Design review of the part shown in the three views and the two pictorial views. Dimensions are in mm from the part's minimum x, y and z. Round coordinates to 2 decimals unless told otherwise and drop trailing zeros. Order: outer loops, then holes, each group sorted by start corner. A loop starts at its lowest first (then second) coordinate and runs counter-clockwise, first axis right, second up.
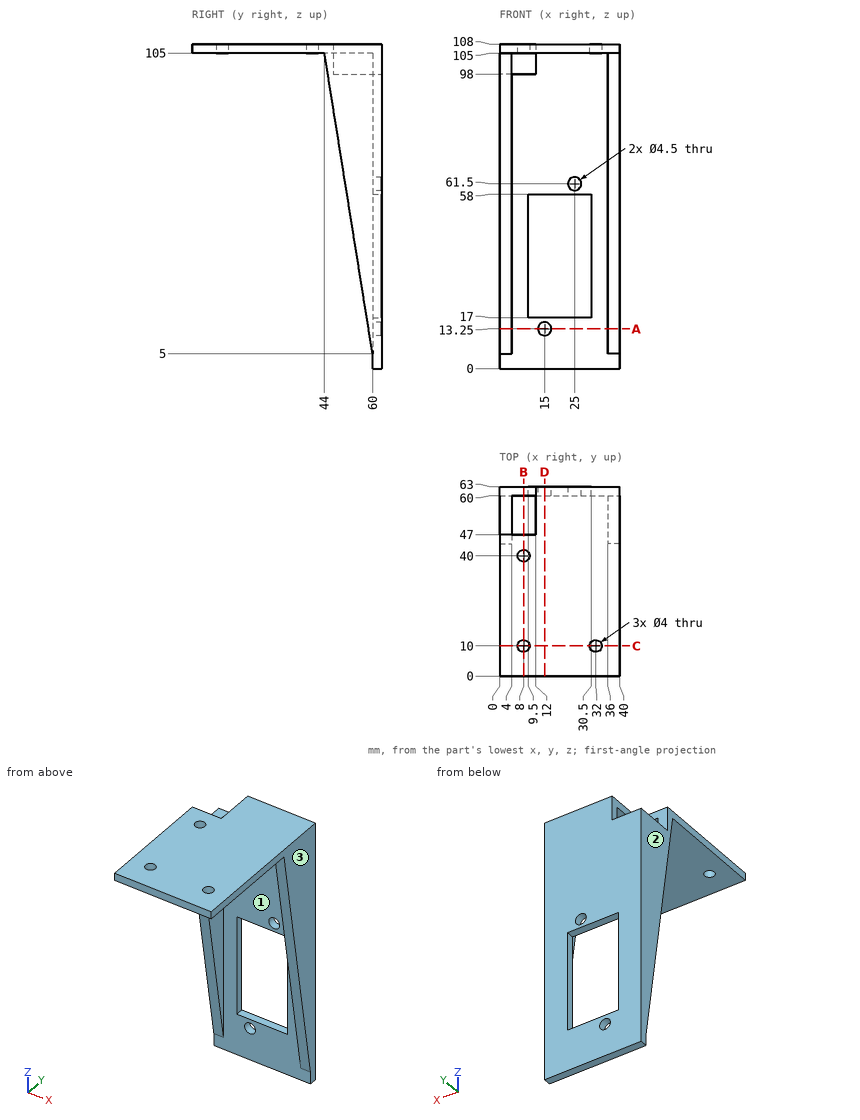
(1) Clearance check with flat-ended pins moving along their axes: P1, Ø3, axis at x = 31, z = 20.5, coming from the -Y side; P2, Ø3, axis at y = 57.5, z = 101, coming from the -X side; P3, Ø11, axis at x = 5.5, z = 104, coming from the +Y side; P4, Ø2.5, axis at x = 25, z = 61.5, coming from the +Y side. State where each tip first meets the part, or that it passes through.
(2) Add section B-B on x = 8. Give the boundary of the cut face in (y, z).
(3) Add section D-D on x = 15. Give the boundary of the cut face in (y, z), plus the area to 4 significant figures.
(4) Draft analysis for pull direction X (two halves, no side actions). For the marked faces 1, 2 and 3, state which applies: pulls with the +X half, pulls with the -X half, needs draft (parallel to the pull), parting line crosses it, or undercut.
(5) Add section A-A on z = 13.25. Give the boundary of the cut face in (x, y), plus the area to 3 significant figures.
(6) Wall thickness on L1, parallel to Z at x = 25, y = 61; L2, parallel to Y at x = 8, z = 106.8; L3, parallel to Z at x = 15, y = 61.85: over which ranges is each line inside the solid? List them lowest first.
(7) Add section C-C on y = 10. Give the boundary of the cut face in (x, z).
Here are the results:
1. P1: stops at y = 60
1. P2: stops at x = 36
1. P3: stops at y = 47
1. P4: passes through
2. outline: (0, 105) - (8, 105) - (8, 108) - (0, 108) - close; (12, 105) - (38, 105) - (38, 108) - (12, 108) - close; (42, 105) - (47, 105) - (47, 108) - (42, 108) - close; (60, 0) - (63, 0) - (63, 98) - (60, 98) - close
3. outline: (0, 105) - (60, 105) - (60, 58) - (63, 58) - (63, 108) - (0, 108) - close; (60, 0) - (63, 0) - (63, 11) - (60, 11) - close; (60, 15.5) - (63, 15.5) - (63, 17) - (60, 17) - close
3. area: 367.5 mm2
4. face 1: undercut
4. face 2: pulls with the -X half
4. face 3: pulls with the +X half
5. outline: (0, 58.68) - (4, 58.68) - (4, 60) - (12.75, 60) - (12.75, 63) - (0, 63) - close; (17.25, 60) - (36, 60) - (36, 58.68) - (40, 58.68) - (40, 63) - (17.25, 63) - close
5. area: 117 mm2
6. L1: z = 0 to 17, 58 to 59.25, 63.75 to 108
6. L2: y = 0 to 8, 12 to 38, 42 to 47
6. L3: z = 0 to 11, 15.5 to 17, 58 to 108
7. outline: (0, 105) - (6, 105) - (6, 108) - (0, 108) - close; (10, 105) - (30, 105) - (30, 108) - (10, 108) - close; (34, 105) - (40, 105) - (40, 108) - (34, 108) - close
